from build123d import *

# Parameters (mm, degrees)
BOSS_EXTRUDE1_DEPTH = 6.35
FILLET1_R           = 2.54
FILLET2_R           = 2.54
FILLET3_R           = 20.32
SKETCH3_R           = 6.35
BOSS_EXTRUDE2_DEPTH = 10.795
FILLET5_R           = 0.762
BOSS_EXTRUDE3_DEPTH = 3.81


with BuildPart() as part:
    # Sketch1 → Boss-Extrude1 (new body)
    with BuildSketch(Plane.XY):
        Polygon((-50.8, 0), (50.8, 0), (50.8, 50.8), (0, 101.6), (-50.8, 50.8), align=None)
    extrude(amount=BOSS_EXTRUDE1_DEPTH)

    # Fillet1
    fillet1_edges = [part.edges().sort_by_distance(p)[0] for p in [
        (50.8, 25.4, 6.35),
        (25.4, 76.2, 6.35),
        (-25.4, 76.2, 6.35),
        (-50.8, 25.4, 6.35),
        (0, 0, 6.35),
    ]]
    fillet(fillet1_edges, radius=FILLET1_R)

    # Fillet2
    fillet2_edges = [part.edges().sort_by_distance(p)[0] for p in [
        (-25.4, 76.2, 0),
        (25.4, 76.2, 0),
        (50.8, 25.4, 0),
        (0, 0, 0),
        (-50.8, 25.4, 0),
    ]]
    fillet(fillet2_edges, radius=FILLET2_R)

    # Fillet3
    # the kernel refuses this fillet: 20.32 mm, written as the material it takes off along each edge
    with BuildSketch(Plane(origin=(30.48, 42.383180413, 6.35), x_dir=(1, 0, 0), z_dir=(0, -1, 0))) as fillet3_piece_1:
        with BuildLine():
            CenterArc((17.78, -2.54), 2.54, 0, 90)
            Line((20.32, -2.54), (20.32, 0))
            Line((20.32, 0), (17.78, 0))
        make_face()
    revolve(axis=Axis((30.48, 42.383180413, 6.35), (0, 0, 1)), revolution_arc=45, mode=Mode.SUBTRACT)
    with BuildSketch(Plane(origin=(0, 72.863180413, 6.35), x_dir=(0.7071067811865475, 0.7071067811865477, 0), z_dir=(0.7071067811865477, -0.7071067811865475, 0))) as fillet3_piece_2:
        with BuildLine():
            CenterArc((17.78, -2.54), 2.54, 0, 90)
            Line((20.32, -2.54), (20.32, 0))
            Line((20.32, 0), (17.78, 0))
        make_face()
    revolve(axis=Axis((0, 72.863180413, 6.35), (0, 0, 1)), revolution_arc=90, mode=Mode.SUBTRACT)
    with BuildSketch(Plane(origin=(-30.48, 42.383180413, 6.35), x_dir=(-0.7071067811865475, 0.7071067811865476, 0), z_dir=(0.7071067811865476, 0.7071067811865475, 0))) as fillet3_piece_3:
        with BuildLine():
            CenterArc((17.78, -2.54), 2.54, 0, 90)
            Line((20.32, -2.54), (20.32, 0))
            Line((20.32, 0), (17.78, 0))
        make_face()
    revolve(axis=Axis((-30.48, 42.383180413, 6.35), (0, 0, 1)), revolution_arc=45, mode=Mode.SUBTRACT)
    with BuildSketch(Plane(origin=(30.48, 42.383180413, 0), x_dir=(0.7071067811865475, 0.7071067811865477, 0), z_dir=(-0.7071067811865477, 0.7071067811865475, 0))) as fillet3_piece_4:
        with BuildLine():
            CenterArc((17.78, -2.54), 2.54, 0, 90)
            Line((20.32, -2.54), (20.32, 0))
            Line((20.32, 0), (17.78, 0))
        make_face()
    revolve(axis=Axis((30.48, 42.383180413, 0), (0, 0, -1)), revolution_arc=45, mode=Mode.SUBTRACT)
    with BuildSketch(Plane(origin=(0, 72.863180413, 0), x_dir=(-0.7071067811865475, 0.7071067811865476, 0), z_dir=(-0.7071067811865476, -0.7071067811865475, 0))) as fillet3_piece_5:
        with BuildLine():
            CenterArc((17.78, -2.54), 2.54, 0, 90)
            Line((20.32, -2.54), (20.32, 0))
            Line((20.32, 0), (17.78, 0))
        make_face()
    revolve(axis=Axis((0, 72.863180413, 0), (0, 0, -1)), revolution_arc=90, mode=Mode.SUBTRACT)
    with BuildSketch(Plane(origin=(-30.48, 42.383180413, 0), x_dir=(-1, 0, 0), z_dir=(0, -1, 0))) as fillet3_piece_6:
        with BuildLine():
            CenterArc((17.78, -2.54), 2.54, 0, 90)
            Line((20.32, -2.54), (20.32, 0))
            Line((20.32, 0), (17.78, 0))
        make_face()
    revolve(axis=Axis((-30.48, 42.383180413, 0), (0, 0, -1)), revolution_arc=45, mode=Mode.SUBTRACT)
    with BuildSketch(Plane(origin=(-50.8, 50.8, 0), x_dir=(0, -1, 0), z_dir=(0, 0, 1))) as fillet3_piece_7:
        with BuildLine():
            CenterArc((FILLET3_R * 0.414213562373, FILLET3_R), FILLET3_R, 225, 45)
            Line((-FILLET3_R * 0.292893218813, FILLET3_R * 0.292893218813), (0, 0))
            Line((0, 0), (FILLET3_R * 0.414213562373, 0))
        make_face()
    extrude(amount=6.35, mode=Mode.SUBTRACT)
    with BuildSketch(Plane(origin=(50.8, 50.8, 0), x_dir=(0, -1, 0), z_dir=(0, 0, 1))) as fillet3_piece_8:
        with BuildLine():
            CenterArc((FILLET3_R * 0.414213562373, -FILLET3_R), FILLET3_R, 90, 45)
            Line((-FILLET3_R * 0.292893218813, -FILLET3_R * 0.292893218813), (0, 0))
            Line((0, 0), (FILLET3_R * 0.414213562373, 0))
        make_face()
    extrude(amount=6.35, mode=Mode.SUBTRACT)
    with BuildSketch(Plane(origin=(0, 101.6, 0), x_dir=(-0.7071067811865476, -0.7071067811865476, 0), z_dir=(0, 0, 1))) as fillet3_piece_9:
        with BuildLine():
            CenterArc((FILLET3_R, FILLET3_R), FILLET3_R, 180, 90)
            Line((0, FILLET3_R), (0, 0))
            Line((0, 0), (FILLET3_R, 0))
        make_face()
    extrude(amount=6.35, mode=Mode.SUBTRACT)

    # Sketch3 → Boss-Extrude2 (add, symmetric)
    with BuildSketch(Plane.XY.offset(6.35)):
        with Locations((0, 71.12)):
            Circle(SKETCH3_R)
    extrude(amount=BOSS_EXTRUDE2_DEPTH, both=True)

    # Fillet5
    fillet5_edges = [part.edges().sort_by_distance(p)[0] for p in [
        (-6.35, 71.12, -4.445),
        (-6.35, 71.12, 17.145),
    ]]
    fillet(fillet5_edges, radius=FILLET5_R)

    # Sketch4 → Boss-Extrude3 (add)
    with BuildSketch(Plane(origin=(0, 0, 0), x_dir=(-1, 0, 0), z_dir=(0, 0, -1))):
        with BuildLine():
            Line((-38.1, 12.7), (38.1, 12.7))
            ThreePointArc((38.1, 12.7), (0, 50.8), (-38.1, 12.7))
        make_face()
    extrude(amount=BOSS_EXTRUDE3_DEPTH)


solid = part.part
Work out the finished part from the listing and answer in its coordinate system (mm). A direction names the side the tool comes from. Coordinates: 2 decimals unless noted, no trailing zeros. Loops run counter-clockwise (first coordinate to the right, second up) from the corner with the lowest first, then second, coordinate; pieces in that order, holes last. Notation, with made-up numbers: M 13,76 L 30,76 A17 cw 30,91 Z; hole C 77.5,33.25 d1. An arc over 180 degrees is marked long. Answer in a Markdown table with one row per item. Add a question column.
1. Consider L1, parallel to Z at x = 31, y = 59.5; L2, parallel to Z at x = -42, y = 56.5; L3, parallel to X at y = 17, z = -3. Determine where each line is inside the solid, lowest interval first.
2. Find section B-B, the plane y = 37. Write down the section's boundary in (x, z), then the cut area to 3 significant figures.
3. A tool of negligible diameter and unlimited length cuts with its end or side. For faces 1 (the flat face through (-1, 57, 0)), 2 (the flat face through (29.8, 71.8, 3.2)), 3 (the cylindrical face through (-1.38, 64.92, 11.44)), 4 (the flat face through (1, 12.7, -2)), from which of +Z, -Z, +X, -X, +Y, -Y can it reach the whole face along a straight path? Write none if from no direction.
4. Find section C-C, the plane z = 15.25. Write down the section's boundary in (x, y).
5. Flat-ended cylindrical pins translate along their axes: P1, Ø8, axis at x = -21, y = 67, coming from the +Z side; P2, Ø2, axis at x = -27.5, z = 8.5, coming from the +Y side; P3, Ø19, axis at x = 7, y = 37.5, coming from the -Z side; P4, Ø5, axis at y = 81.5, z = 4, coming from the -X side. Find the tip coordinate at first contact, or state that the pin passes through.
6. Find section A-A, the plane x = 0. Write down the section's boundary in (y, z) (3 decimals), then the cut area to 3 significant figures.
Reported:
| question | item | result |
|---|---|---|
| 1 | L1 | z = 0 to 6.35 |
| 1 | L2 | z = 0.02 to 6.33 |
| 1 | L3 | x = -37.86 to 37.86 |
| 2 | outline | M -50.8,2.54 A2.54 ccw -48.26,0 L -29.34,0 L -29.34,-3.81 L 29.34,-3.81 L 29.34,0 L 48.26,0 A2.54 ccw 50.8,2.54 L 50.8,3.81 A2.54 ccw 48.26,6.35 L -48.26,6.35 A2.54 ccw -50.8,3.81 Z |
| 2 | area | 863 mm^2 |
| 3 | face 1 | -Z |
| 3 | face 2 | +Z, -Z, +X, +Y |
| 3 | face 3 | +Z |
| 3 | face 4 | -Z, +X, -X, -Y |
| 4 | outline | C 0,71.12 d12.7 |
| 5 | P1 | stops at z = 6.35 |
| 5 | P2 | passes through |
| 5 | P3 | stops at z = -3.81 |
| 5 | P4 | stops at x = -22.6 |
| 6 | outline | M 0,2.54 A2.54 ccw 2.54,0 L 12.7,0 L 12.7,-3.81 L 50.8,-3.81 L 50.8,0 L 64.77,0 L 64.77,-3.683 A0.762 ccw 65.532,-4.445 L 76.708,-4.445 A0.762 ccw 77.47,-3.683 L 77.47,0 L 90.643,0 A2.54 ccw 93.183,2.54 L 93.183,3.81 A2.54 ccw 90.643,6.35 L 77.47,6.35 L 77.47,16.383 A0.762 ccw 76.708,17.145 L 65.532,17.145 A0.762 ccw 64.77,16.383 L 64.77,6.35 L 2.54,6.35 A2.54 ccw 0,3.81 Z |
| 6 | area | 924 mm^2 |
